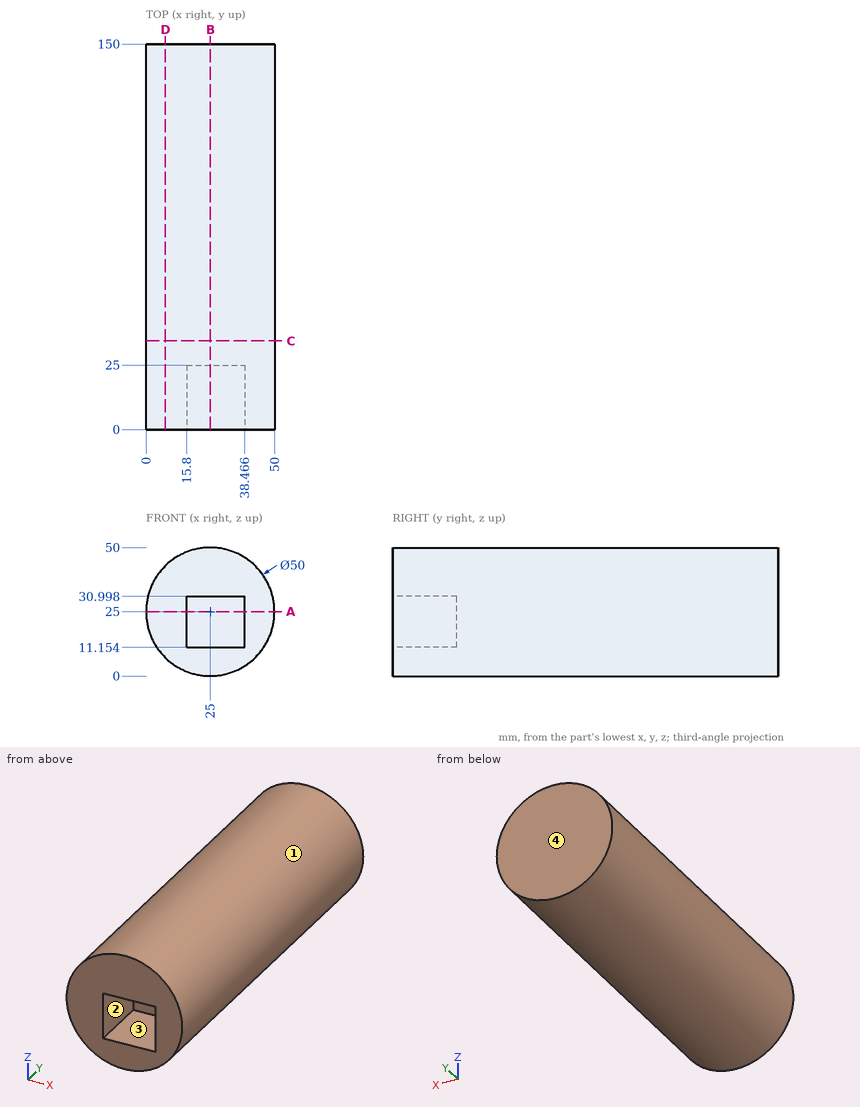
For this review, use the dimensioned drawing (mm, ordinates from the lowest corner) and the shaded views. Coordinates: 2 decimals unless noted, no trailing zeros. Loops run counter-clockwise (first coordinate to the right, second up) from the corner with the lowest first, then second, coordinate; pieces in that order, holes last. Notation, with made-up numbers: (30, 6.25) -> (79, 6.25) arc R21 cw to (79, 36.25) -> close; hole circle Ø9 at (-15, 86). An arc over 180 degrees is marked (long way). Return JSON: item names as keys, results as strings. Group by question number.
(1) Consider section D-D, the plane x = 7.5. Give the boundary of the cut face in (y, z).
(2) For pin 1 Ø7 at (x, y) = (30, 7.5) entering from +Z (1 decimal); pin 2 Ø1 at (y, z) = (34, 27) entering from +X (1 decimal); pin 3 Ø6 at (x, z) = (27.5, 23.5) entering from -Y, all flat-tipped, find the tip position at first contact; note any pin that passes through.
(3) Mouldability with a two-part tool opening along X and no side actions: class the marked faces 1, 2, 3 and 4 as pulls with the +X half, pulls with the -X half, needs draft (parallel to the pull), parting line crosses it, or undercut.
(4) Consider section C-C, the plane y = 34.5. Give the boundary of the cut face in (x, z), plus the area to 3 significant figures.
(5) Consider section B-B, the plane x = 25. Give the boundary of the cut face in (y, z), plus the area to 3 significant figures.
(6) To check wall thickness, follow L1, parallel to X at y = 78.5, z = 26; L2, parallel to Z at x = 26, y = 18; L3, parallel to Y at x = 16, z = 29. State the ranges of each line that lie inside material, in increasing order.
(7) Consider section A-A, the plane z = 25. Give the boundary of the cut face in (x, y), plus the area to 3 significant figures.
Results below:
{
 "1": {"outline": "(0, 7.15) -> (150, 7.15) -> (150, 42.85) -> (0, 42.85) -> close"},
 "2": {"pin 1": "stops at z = 50", "pin 2": "stops at x = 50", "pin 3": "stops at y = 25"},
 "3": {"face 1": "parting line crosses it", "face 2": "undercut", "face 3": "undercut", "face 4": "needs draft"},
 "4": {"outline": "circle Ø50 at (25, 25)", "area": "1,960 mm2"},
 "5": {"outline": "(0, 0) -> (150, 0) -> (150, 50) -> (0, 50) -> (0, 31) -> (25, 31) -> (25, 11.15) -> (0, 11.15) -> close", "area": "7,000 mm2"},
 "6": {"L1": "x = 0.02 to 49.98", "L2": "z = 0.02 to 11.15, 31 to 49.98", "L3": "y = 25 to 150"},
 "7": {"outline": "(0, 0) -> (15.8, 0) -> (15.8, 25) -> (38.47, 25) -> (38.47, 0) -> (50, 0) -> (50, 150) -> (0, 150) -> close", "area": "6,930 mm2"}
}
